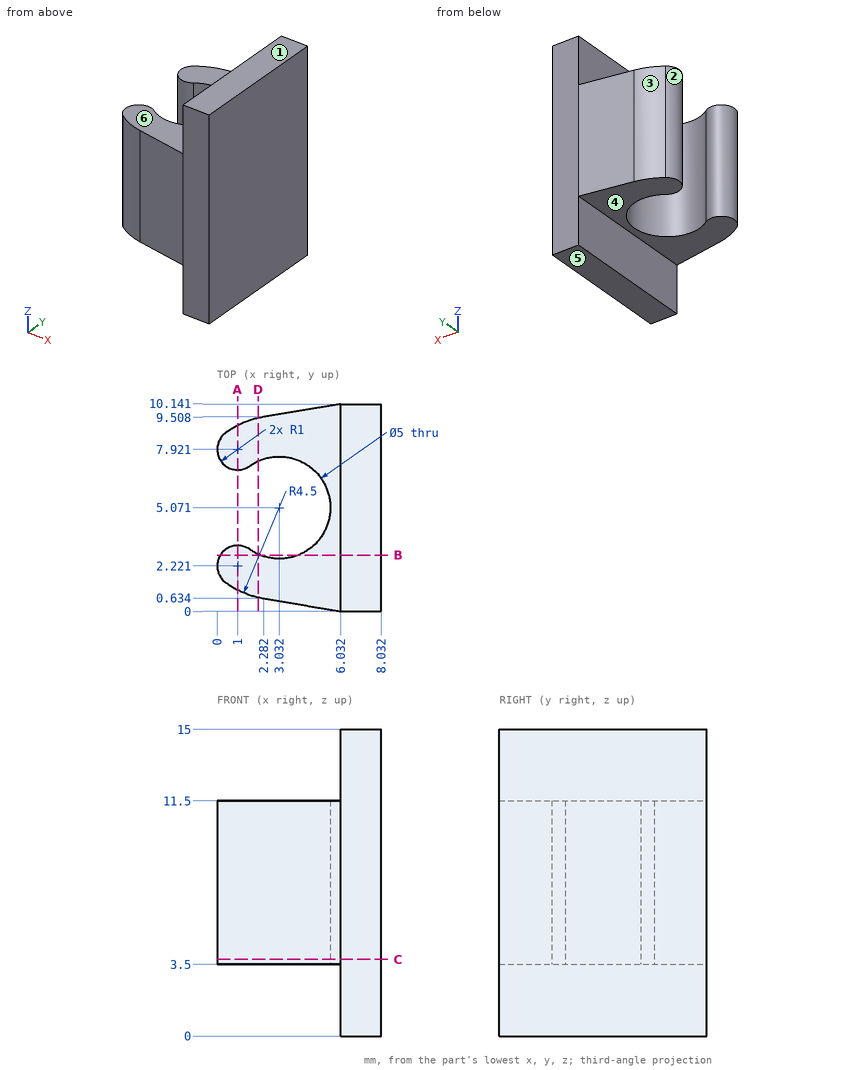
Source: three-view drawing plus pictorial views. Frame: mm from the lowest corner of the part. A direction names the side the tool comes from. Coordinates: 2 decimals unless noted, no trailing zeros. Order: outer loops, then holes, each group sorted by start corner. A loop starts at its lowest first (then second) coordinate and runs counter-clockwise, first axis right, second up.
Item 1: Cut plane C-C (z = 3.75). Return loops of the section in (x, y) (1 decimal), plus the area to 3 significant figures.
Output values:
outline: (0.4, 1.4) arc R4.5 ccw to (2.3, 0.6) - (6, 0) - (8, 0) - (8, 10.1) - (6, 10.1) - (2.3, 9.5) arc R4.5 ccw to (0.4, 8.7) arc R1 ccw to (1.6, 7.1) arc R2.5 cw (long way) to (1.6, 3) arc R1 ccw to start
area: 51.2 mm2
Item 2: Cut plane A-A (x = 1). Return loops of the section in (y, z) (1 decimal).
Output values:
outline: (1.1, 3.5) - (3.2, 3.5) - (3.2, 11.5) - (1.1, 11.5) - close; (6.9, 3.5) - (9.1, 3.5) - (9.1, 11.5) - (6.9, 11.5) - close
Item 3: Cut plane B-B (y = 2.75). Return loops of the section in (x, z).
Output values:
outline: (0.15, 3.5) - (2.1, 3.5) - (2.1, 11.5) - (0.15, 11.5) - close; (3.96, 3.5) - (6.03, 3.5) - (6.03, 0) - (8.03, 0) - (8.03, 15) - (6.03, 15) - (6.03, 11.5) - (3.96, 11.5) - close
Item 4: Pull-direction query (X, two-part tool) for the marked faces 1, 2 and 3; classes: pulls with the +X half, pulls with the -X half, needs draft (parallel to the pull), parting line crosses it, or undercut.
Output values:
face 1: needs draft
face 2: undercut
face 3: pulls with the -X half
Item 5: First-contact query: P1, Ø1.8, axis at x = 1.5, y = 3.5, coming from the -Z side. Flat tip, straight axial feed; report the tip coordinate or a pass-through.
Output values:
P1: stops at z = 3.5
Item 6: Material intervals for line 1 (Y direction, x = 4.75, z = 10.5) (1 decimal); line 2 (X direction, y = 3.25, z = 12.25); line 3 (Z direction, x = 2.75, y = 9.5), sorted ascending.
Output values:
line 1: y = 0.2 to 3.3, 6.9 to 9.9
line 2: x = 6.03 to 8.03
line 3: z = 3.5 to 11.5
Item 7: Set-up query: the marked faces 4, 5 and 6. Return all of +Z, -Z, +X, -X, +Y, -Y with unobstructed straight access to the full face (end or side cutting, diameter ignored); none if empty.
Output values:
face 4: -Z, -X, +Y, -Y
face 5: -Z, +X, -X, +Y, -Y
face 6: +Z, -X, +Y, -Y
Item 8: Cut plane D-D (x = 2). Return loops of the section in (y, z).
Output values:
outline: (0.69, 3.5) - (2.79, 3.5) - (2.79, 11.5) - (0.69, 11.5) - close; (7.35, 3.5) - (9.45, 3.5) - (9.45, 11.5) - (7.35, 11.5) - close
